from build123d import *

# Parameters (mm, degrees)
SKETCH1_W           = 254
SKETCH1_H           = 152.4
BOSS_EXTRUDE1_DEPTH = 12.7
SKETCH4_OUTSIDE_W   = 315.296
SKETCH4_OUTSIDE_H   = 213.696
CUT_EXTRUDE1_DEPTH  = 13.7
BOSS_EXTRUDE2_DEPTH = 6.35
BOSS_EXTRUDE3_START = 6.35
BOSS_EXTRUDE3_DEPTH = 6.35
FILLET1_R           = 1.27
CUT_EXTRUDE3_DEPTH  = 13.7000001


with BuildPart() as part:
    # Sketch1 → Boss-Extrude1 (new body)
    with BuildSketch(Plane(origin=(0, 0, 0), x_dir=(1, 0, 0), z_dir=(0, 1, 0))):
        Rectangle(SKETCH1_W, SKETCH1_H)
    extrude(amount=BOSS_EXTRUDE1_DEPTH)

    # Sketch4 outside → Cut-Extrude1 (cut, through all)
    with BuildSketch(Plane.XZ):
        Rectangle(SKETCH4_OUTSIDE_W, SKETCH4_OUTSIDE_H)
        with BuildLine():
            Line((48.514, 25.621286072), (48.514, 38.735))
            ThreePointArc((48.514, 38.735), (45.649797213, 45.649797213), (38.735, 48.514))
            Line((38.735, 48.514), (25.621286072, 48.514))
            ThreePointArc((25.621286072, 48.514), (0, 54.864), (-25.621286072, 48.514))
            Line((-25.621286072, 48.514), (-38.735, 48.514))
            ThreePointArc((-38.735, 48.514), (-45.649797213, 45.649797213), (-48.514, 38.735))
            Line((-48.514, 38.735), (-48.514, 25.621286072))
            ThreePointArc((-48.514, 25.621286072), (-54.864, 0), (-48.514, -25.621286072))
            Line((-48.514, -25.621286072), (-48.514, -38.735))
            ThreePointArc((-48.514, -38.735), (-45.649797213, -45.649797213), (-38.735, -48.514))
            Line((-38.735, -48.514), (-25.621286072, -48.514))
            ThreePointArc((-25.621286072, -48.514), (0, -54.864), (25.621286072, -48.514))
            Line((25.621286072, -48.514), (38.735, -48.514))
            ThreePointArc((38.735, -48.514), (45.649797213, -45.649797213), (48.514, -38.735))
            Line((48.514, -38.735), (48.514, -25.621286072))
            ThreePointArc((48.514, -25.621286072), (54.864, 0), (48.514, 25.621286072))
        make_face(mode=Mode.SUBTRACT)
        with BuildLine():
            Line((45.339, 24.821921763), (45.339, 38.735))
            ThreePointArc((45.339, 38.735), (43.404733183, 43.404733183), (38.735, 45.339))
            Line((38.735, 45.339), (24.821921763, 45.339))
            ThreePointArc((24.821921763, 45.339), (0, 51.689), (-24.821921763, 45.339))
            Line((-24.821921763, 45.339), (-38.735, 45.339))
            ThreePointArc((-38.735, 45.339), (-43.404733183, 43.404733183), (-45.339, 38.735))
            Line((-45.339, 38.735), (-45.339, 24.821921763))
            ThreePointArc((-45.339, 24.821921763), (-51.689, 0), (-45.339, -24.821921763))
            Line((-45.339, -24.821921763), (-45.339, -38.735))
            ThreePointArc((-45.339, -38.735), (-43.404733183, -43.404733183), (-38.735, -45.339))
            Line((-38.735, -45.339), (-24.821921763, -45.339))
            ThreePointArc((-24.821921763, -45.339), (0, -51.689), (24.821921763, -45.339))
            Line((24.821921763, -45.339), (38.735, -45.339))
            ThreePointArc((38.735, -45.339), (43.404733183, -43.404733183), (45.339, -38.735))
            Line((45.339, -38.735), (45.339, -24.821921763))
            ThreePointArc((45.339, -24.821921763), (51.689, 0), (45.339, 24.821921763))
        make_face()
    extrude(amount=-CUT_EXTRUDE1_DEPTH, mode=Mode.SUBTRACT)

    # Sketch5 → Boss-Extrude2 (add)
    with BuildSketch(Plane(origin=(0, 0, 0), x_dir=(1, 0, 0), z_dir=(0, 1, 0))):
        with BuildLine():
            Line((54.495284163, 6.35), (104.775, 6.35))
            Line((104.775, 6.35), (92.075, -6.35))
            Line((92.075, -6.35), (54.495284163, -6.35))
            ThreePointArc((54.495284163, -6.35), (54.864, 0), (54.495284163, 6.35))
        make_face()
        with BuildLine():
            Line((-92.075, -6.35), (-54.495284163, -6.35))
            ThreePointArc((-54.495284163, -6.35), (-54.864, 0), (-54.495284163, 6.35))
            Line((-54.495284163, 6.35), (-104.775, 6.35))
            Line((-104.775, 6.35), (-92.075, -6.35))
        make_face()
    extrude(amount=BOSS_EXTRUDE2_DEPTH)

    # Sketch6 → Boss-Extrude3 (add)
    with BuildSketch(Plane(origin=(0, 0, 0), x_dir=(1, 0, 0), z_dir=(0, 1, 0)).offset(BOSS_EXTRUDE3_START)):
        with BuildLine():
            Line((53.373855922, 12.7), (111.125, 12.7))
            Line((111.125, 12.7), (73.025, -25.4))
            Line((73.025, -25.4), (48.630222043, -25.4))
            ThreePointArc((48.630222043, -25.4), (54.443644996, -6.778496559), (53.373855922, 12.7))
        make_face()
        with BuildLine():
            Line((-73.025, -25.4), (-48.630222043, -25.4))
            ThreePointArc((-48.630222043, -25.4), (-54.443644996, -6.778496559), (-53.373855922, 12.7))
            Line((-53.373855922, 12.7), (-111.125, 12.7))
            Line((-111.125, 12.7), (-73.025, -25.4))
        make_face()
    extrude(amount=BOSS_EXTRUDE3_DEPTH)

    # Fillet1
    fillet1_edges = [part.edges().sort_by_distance(p)[0] for p in [
        (51.689, 0, 0),
        (45.339, 0, 31.778460881),
        (43.404733183, 0, 43.404733183),
        (31.778460881, 0, 45.339),
        (0, 0, 51.689),
        (-31.778460881, 0, 45.339),
        (-43.404733183, 0, 43.404733183),
        (-45.339, 0, 31.778460881),
        (-51.689, 0, 0),
        (-45.339, 0, -31.778460881),
        (-43.404733183, 0, -43.404733183),
        (-31.778460881, 0, -45.339),
        (0, 0, -51.689),
        (31.778460881, 0, -45.339),
        (43.404733183, 0, -43.404733183),
        (45.339, 0, -31.778460881),
    ]]
    fillet(fillet1_edges, radius=FILLET1_R)

    # Sketch9 → Cut-Extrude3 (cut, through all)
    with BuildSketch(Plane(origin=(0, 12.7, 0), x_dir=(1, 0, 0), z_dir=(0, 1, 0))):
        with BuildLine():
            Line((38.735, -48.514), (35.814, -48.514))
            ThreePointArc((35.814, -48.514), (44.794256121, -44.794256121), (48.514, -35.814))
            Line((48.514, -35.814), (48.514, -38.735))
            ThreePointArc((48.514, -38.735), (45.649797213, -45.649797213), (38.735, -48.514))
        make_face()
        with BuildLine():
            Line((-48.514, -35.814), (-48.514, -38.735))
            ThreePointArc((-48.514, -38.735), (-45.649797213, -45.649797213), (-38.735, -48.514))
            Line((-38.735, -48.514), (-35.814, -48.514))
            ThreePointArc((-35.814, -48.514), (-44.794256121, -44.794256121), (-48.514, -35.814))
        make_face()
    extrude(amount=-CUT_EXTRUDE3_DEPTH, mode=Mode.SUBTRACT)


solid = part.part
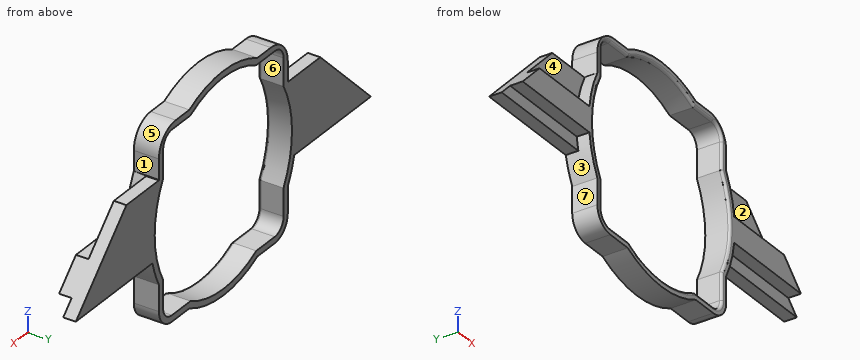
Work out the finished part from the listing and answer in its coordinate system (mm). Face numbers are marked on the shaded views. A direction names the side the tool comes from. Round coordinates to 2 decimals unless told otherwise and drop trailing zeros. Order: outer loops, then holes, each group sorted by start corner. A loop starts at its lowest first (then second) coordinate and runs counter-clockwise, first axis right, second up. Notation, with made-up numbers: M 56.5,17 L 114.5,17 A34 ccw 114.5,47 Z; hole C 68.25,63 d11. An arc over 180 degrees is marked long. Put each result on its own line as item: value. Start each with the question number.
Q1. Section B-B, the plane z = 28 is taken. Write down the section's boundary in (x, y), and give its area (3 significant figures).
Q2. Section A-A, the plane x = -32.5 is taken. Write down the section's boundary in (y, z).
Q3. For a pull along X with two mould halves and no side action, classify the marked faces 5, 6 and 7 as pulls with the +X half, pulls with the -X half, needs draft (parallel to the pull), parting line crosses it, or undercut.
Q4. Straight lines are drawn through the part: L1, parallel to X at y = 1.75, z = -28; L2, parallel to X at y = 9, z = -47; L3, parallel to Z at x = -72.5, y = 5.75. For each, find the intervals that lie inside material, in ascending order. Write a range as [from, to].
Q5. Flat-ended cylindrical pins translate along their axes: pin 1 (3 mm diameter, centred on y = 7, z = 40, fed in from +X); pin 2 (3 mm diameter, centred on y = 8, z = 20, fed in from +X) (3 decimals); pin 3 (5 mm diameter, centred on y = 7, z = 25, fed in from -X) (3 decimals). Find the tip coordinate at first contact, or state that the pin passes through.
Q6. A tool of negligible diameter and unlimited length cuts with its end or side. For the marked faces 1, 2, 3 and 4, from which of +Z, -Z, +X, -X, +Y, -Y can it reach the whole face along a straight path? Write none if from no direction.
Findings below:
1. outline: M -48.51,0 L -46.61,0 A1.27 ccw -45.34,1.27 L -45.34,12.7 L -48.51,12.7 Z; M 45.34,1.27 A1.27 ccw 46.61,0 L 48.51,0 L 48.51,12.7 L 45.34,12.7 Z
1. area: 80.0 mm^2
2. outline: M 0,-48.51 L 12.7,-48.51 L 12.7,-45.34 L 1.27,-45.34 A1.27 ccw 0,-46.61 Z; M 0,46.61 A1.27 ccw 1.27,45.34 L 12.7,45.34 L 12.7,48.51 L 0,48.51 Z
3. face 5: pulls with the +X half
3. face 6: undercut
3. face 7: pulls with the -X half
4. L1: x = [-48.51, -45.34], [45.34, 48.51]
4. L2: x = [-43.96, -21.51], [21.51, 43.96]
4. L3: z = [-6.35, 6.35]
5. pin 1: stops at x = 48.23
5. pin 2: stops at x = 79.925
5. pin 3: stops at x = -75.925
6. face 1: +Z, +X, +Y, -Y
6. face 2: +Z, +X, -Y
6. face 3: -Z, -X, -Y
6. face 4: +Z, -X, -Y
